Drawing for the job (mm, zero at the part's lowest x, y, z). A direction names the side the tool comes from. Give positions to 0.01 mm unless a question says otherwise; leave off trailing zeros. Write each loop counter-clockwise with the first axis right and the second up, starting at its lowest first coordinate (ties: lowest second). Pieces come first, ordered by that corner, then holes.
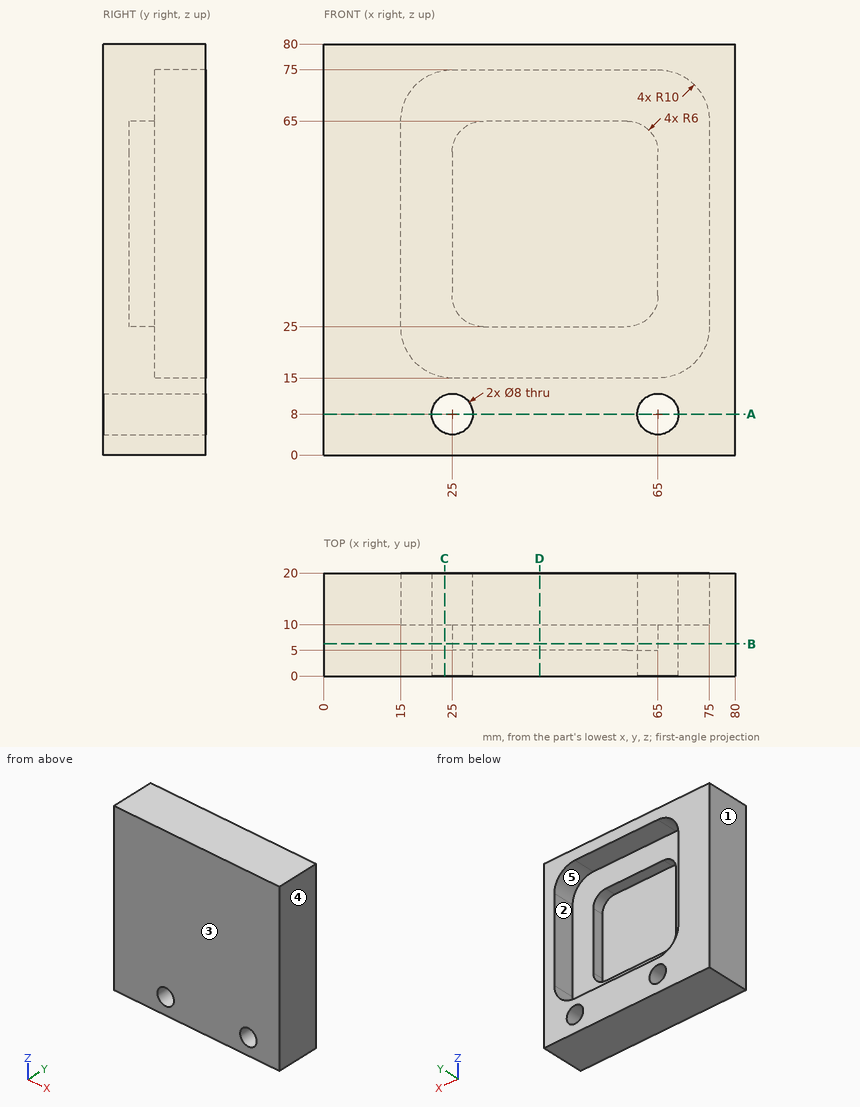
1. Slice it at D-D, the plane x = 42. Write the cut outline in (y, z), and give its area (3 significant figures).
Calculated:
outline: (0, 0) - (20, 0) - (20, 15) - (10, 15) - (10, 25) - (5, 25) - (5, 65) - (10, 65) - (10, 75) - (20, 75) - (20, 80) - (0, 80) - close
area: 800 mm2
2. Probe probe 1 along Z at (x, y) = (65, 15.75); probe 2 along X at (y, z) = (9.75, 40); probe 3 along Y at (x, z) = (71, 43). List the from-to ranges inside material, lowest first.
Calculated:
probe 1: z = 0 to 4, 12 to 15, 75 to 80
probe 2: x = 0 to 25, 65 to 80
probe 3: y = 0 to 10
3. Slice it at A-A, the plane z = 8. Write the cut outline in (x, y), and give its area (3 significant figures).
Calculated:
outline: (0, 0) - (21, 0) - (21, 20) - (0, 20) - close; (29, 0) - (61, 0) - (61, 20) - (29, 20) - close; (69, 0) - (80, 0) - (80, 20) - (69, 20) - close
area: 1,280 mm2
4. Which spindle directions (+Z, -Z, +X, -X, +Y, -Y) get a long thin tool onto all of the face, cutting with end or side? Do the marked faces 1 and 2. Say none if no direction does.
Calculated:
face 1: +Z, -Z, -X, +Y, -Y
face 2: +Y
5. Slice it at B-B, the plane y = 6.25. Write the cut outline in (x, z).
Calculated:
outline: (0, 0) - (80, 0) - (80, 80) - (0, 80) - close; hole circle Ø8 at (25, 8); hole (25, 31) arc R6 ccw to (31, 25) - (59, 25) arc R6 ccw to (65, 31) - (65, 59) arc R6 ccw to (59, 65) - (31, 65) arc R6 ccw to (25, 59) - close; hole circle Ø8 at (65, 8)
6. Slice it at C-C, the plane x = 23.5. Write the cut outline in (y, z).
Calculated:
outline: (0, 0) - (20, 0) - (20, 4.29) - (0, 4.29) - close; (0, 11.71) - (20, 11.71) - (20, 15.11) - (10, 15.11) - (10, 74.89) - (20, 74.89) - (20, 80) - (0, 80) - close
7. Pull direction X, two halves, no side cores. Call the marked faces 3, 4 and 5: +X half, -X half, draft (parallel to the pull), parting line (faces both ways), or undercut.
Calculated:
face 3: draft
face 4: +X half
face 5: undercut
8. Pin check, flat tip, straight feed: P1, Ø18, axis at x = 46, z = 35, coming from the +Y side. Stop position of the tip, or through.
Calculated:
P1: stops at y = 5
